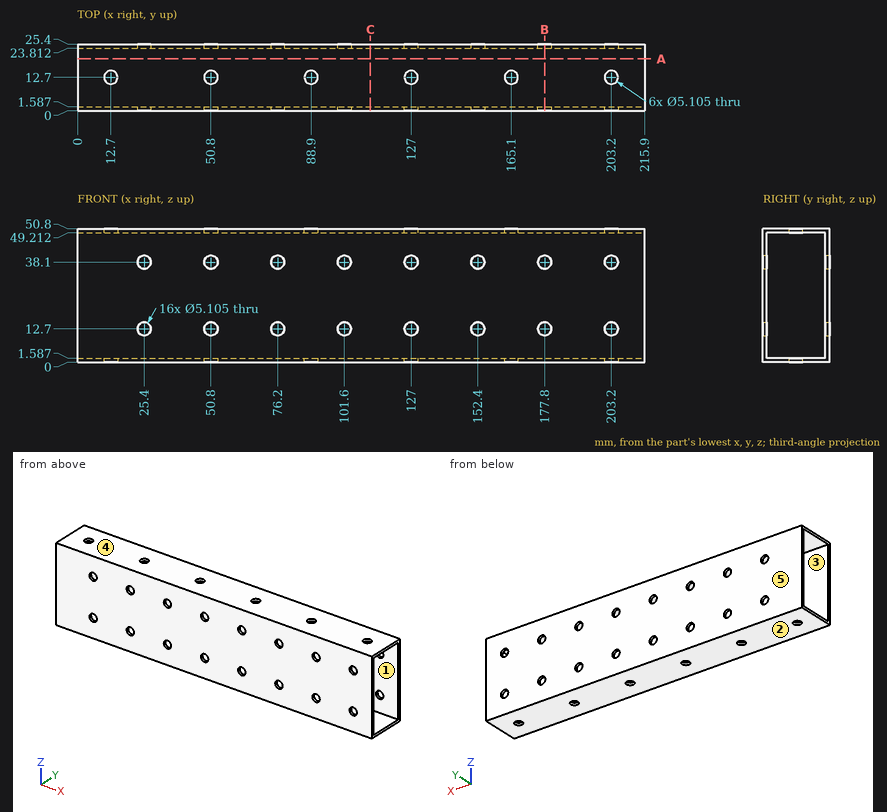
Can you work these out from the drawing? Everything is in mm from the part's minimum corner. A direction names the side the tool comes from. Coordinates: 2 decimals unless noted, no trailing zeros. Loops run counter-clockwise (first coordinate to the right, second up) from the corner with the lowest first, then second, coordinate; pieces in that order, holes last.
1) For pin 1 (12 mm diameter, centred on y = 13, z = 15, fed in from -X), with a flat end and sliding along its axis, tell me the tip position at first contact or that it passes through.
2) Imagine slicing it at C-C on x = 111.5. List the corners of the cut face in (y, z) for me, plus the area to 3 significant figures.
3) Thinking about a two-plate mould opening in Y: for the marked faces 3, 4 and 5, which applies, pulls with the +Y half, pulls with the -Y half, needs draft (parallel to the pull), parting line crosses it, or undercut?
4) Imagine slicing it at B-B on x = 177.8. List the corners of the cut face in (y, z) for me.
5) Which directions (+Z, -Z, +X, -X, +Y, -Y) give clear straight access to the entire face, cutting with the end or side of a thin tool? Please do the marked faces 1 and 2.
6) Imagine slicing it at A-A on y = 19.75. List the corners of the cut face in (x, z) for me.
7) I need wall thicknesses on probe 1 along Z at (x, y) = (152.4, 0.6); probe 2 along Y at (x, z) = (116.5, 2); probe 3 along Y at (x, z) = (165.1, 49.75). Which ranges of each line are inside material? Lowest first, please.
Completed:
1. pin 1: passes through
2. outline: (0, 0) - (25.4, 0) - (25.4, 50.8) - (0, 50.8) - close; hole (1.59, 1.59) - (23.81, 1.59) - (23.81, 49.21) - (1.59, 49.21) - close
2. area: 232 mm2
3. face 3: undercut
3. face 4: needs draft
3. face 5: pulls with the +Y half
4. outline: (0, 0) - (25.4, 0) - (25.4, 10.15) - (23.81, 10.15) - (23.81, 1.59) - (1.59, 1.59) - (1.59, 10.15) - (0, 10.15) - close; (0, 15.25) - (1.59, 15.25) - (1.59, 35.55) - (0, 35.55) - close; (0, 40.65) - (1.59, 40.65) - (1.59, 49.21) - (23.81, 49.21) - (23.81, 40.65) - (25.4, 40.65) - (25.4, 50.8) - (0, 50.8) - close; (23.81, 15.25) - (25.4, 15.25) - (25.4, 35.55) - (23.81, 35.55) - close
5. face 1: +X, -X
5. face 2: -Z, +X, -X, +Y, -Y
6. outline: (0, 0) - (215.9, 0) - (215.9, 1.59) - (0, 1.59) - close; (0, 49.21) - (215.9, 49.21) - (215.9, 50.8) - (0, 50.8) - close
7. probe 1: z = 0 to 10.15, 15.25 to 35.55, 40.65 to 50.8
7. probe 2: y = 0 to 1.59, 23.81 to 25.4
7. probe 3: y = 0 to 10.15, 15.25 to 25.4
